Autodesk Inventor part; units mm, degrees
ref_plane "YZ Plane" through (0, 0, 0) normal (1, 0, 0) x (0, 1, 0)
ref_plane "XZ Plane" through (0, 0, 0) normal (0, 1, 0) x (-1, 0, 0)
ref_plane "XY Plane" through (0, 0, 0) normal (0, 0, 1) x (1, 0, 0)
sketch "Skizze1" plane through (0, 0, 0) normal (0, 0, 1) x (1, 0, 0)
  line L0 (0, -63.8443) -> (0, 15.5659)
  line L1 (-61.5828, 0) -> (61.5828, 0)
  line L2 (-13.5, -52.5) -> (13.5, -52.5)
  line L3 (13.5, -52.5) -> (34.4955, -29.2204)
  line L4 (-13.5, -52.5) -> (-34.4955, -29.2204)
  arc A0 (-21.5, 0) -> (-34.4955, -29.2204) centre (-21.5, -17.5) ccw
  arc A1 (34.4955, -29.2204) -> (21.5, 0) centre (21.5, -17.5) ccw
  line L5 (-21.5, 0) -> (21.5, 0)
  point P0 (0, 0)
  dimension "d0" = 43
  dimension "d1" = 27
  dimension "d2" = 35
  dimension "d3" = 17.5
extrude "Extrusion1" add sketch "Skizze1" along normal blind 5
sketch "Skizze2" plane through (0, 0, 5) normal (0, 0, 1) x (1, 0, 0)
  line L0 (-61.5828, 0) -> (61.5828, 0)
  line L1 (0, -63.8443) -> (0, 15.5659)
  arc A0 (-21.5, 0) -> (-34.4955, -29.2204) centre (-21.5, -17.5) ccw
  circle A1 centre (-21.5, -17.5) radius 4
  arc A2 (34.4955, -29.2204) -> (21.5, 0) centre (21.5, -17.5) ccw
  circle A3 centre (21.5, -17.5) radius 10
  circle A4 centre (-11, -42.5) radius 1.7
  circle A5 centre (11, -42.5) radius 1.7
  line L2 (-13.5, -52.5) -> (13.5, -52.5)
  point P0 (0, 0)
  dimension "d7" = 8
  dimension "d8" = 20
  dimension "d9" = 3.4
  dimension "d10" = 3.4
  dimension "d11" = 10
  dimension "d12" = 22
extrude "Extrusion2" cut sketch "Skizze2" against normal up to next
sketch "Skizze3" plane through (0, 0, 5) normal (0, 0, 1) x (1, 0, 0)
  arc A0 (-21.5, 0) -> (-34.4955, -29.2204) centre (-21.5, -17.5) ccw construction
  circle A1 centre (-21.5, -17.5) radius 15 construction
  line L0 (-21.5, -2.5) -> (-21.5, -32.5) construction
  point P0 (0, 0)
  dimension "d15" = 30
hole "Bohrung1" at (-21.5, -32.5, 5) direction (0, 0, -1) diameter 3.5 end up to surface
pattern_circular "Runde Anordnung1" count 3 over 360 about axis through (-21.5, -17.5, 5) along (0, 0, -1) of "Bohrung1"
sketch "Skizze4" plane through (0, 0, 5) normal (0, 0, 1) x (1, 0, 0)
  arc A0 (34.4955, -29.2204) -> (21.5, 0) centre (21.5, -17.5) ccw construction
  circle A1 centre (21.5, -17.5) radius 14 construction
  line L0 (21.5, -3.5) -> (21.5, -31.5) construction
  point P0 (0, 0)
  dimension "d26" = 28
hole "Bohrung2" at (21.5, -31.5, 5) direction (0, 0, -1) diameter 2.459 end up to surface
pattern_circular "Runde Anordnung2" count 6 over 360 about axis through (21.5, -17.5, 5) along (0, 0, -1) of "Bohrung2"
properties part number "Zylinderplatte"
Can you work these out from the model? Positions are in its coordinate system, mm. Round coordinates to 2 decimals unless told otherwise and drop trailing zeros. Loops run counter-clockwise (first coordinate to the right, second up) from the corner with the lowest first, then second, coordinate; pieces in that order, holes last. Notation, with made-up numbers: (80.25, -35.5) -> (110.25, -35.5) arc R11 cw to (110.25, -23.5) -> close; hole circle Ø2 at (30, 24.25). An arc over 180 degrees is marked (long way). Answer in a Markdown table with one row per item.
Item 1: Suppose I cut it at A-A, the plane y = -18.5. List the corners of the cut face in (x, z) for me.
Answer block:
| item | result |
|---|---|
| outline | (-38.97, 0) -> (-25.37, 0) -> (-25.37, 5) -> (-38.97, 5) -> close; (-17.63, 0) -> (11.55, 0) -> (11.55, 5) -> (-17.63, 5) -> close; (31.45, 0) -> (38.97, 0) -> (38.97, 5) -> (31.45, 5) -> close |
Item 2: Suppose I cut it at B-B, the plane x = 23.5. List the corners of the cut face in (y, z) for me.
Answer block:
| item | result |
|---|---|
| outline | (-41.41, 0) -> (-27.3, 0) -> (-27.3, 5) -> (-41.41, 5) -> close; (-7.7, 0) -> (-0.11, 0) -> (-0.11, 5) -> (-7.7, 5) -> close |
Item 3: We'd pull the mould along Y, two halves only. Please class faces 1 (the flat face through (-1, -26, 5)), 2 (the flat face through (0, -52.5, 2)), 3 (the cylindrical face through (34.715, -11.067, 2.465)): released by +Y, released by -Y, zero draft, split by the parting line, or undercut.
Answer block:
| item | result |
|---|---|
| face 1 | zero draft |
| face 2 | released by -Y |
| face 3 | undercut |
Item 4: If I drill on probe 1 along X at (y, z) = (-17, 0.8); probe 2 along X at (y, z) = (-10, 1.8); probe 3 along Y at (x, z) = (21, 2.9), over which ranges is the centre line in solid material (lowest first)?
Answer block:
| item | result |
|---|---|
| probe 1 | -38.99 to -25.47, -17.53 to 11.51, 31.49 to 38.99 |
| probe 2 | -37.31 to -36.24, -32.74 to -10.26, -6.76 to 8.25, 10.5 to 14.89, 28.11 to 32.5, 34.75 to 37.31 |
| probe 3 | -44.18 to -32.62, -30.38 to -27.49, -7.51 to -4.62, -2.38 to 0 |
Item 5: Suppose I cut it at D-D, the plane y = -10.5. List the corners of the cut face in (x, z) for me, plus the area to 3 significant figures.
Answer block:
| item | result |
|---|---|
| outline | (-37.54, 0) -> (-36.17, 0) -> (-36.17, 5) -> (-37.54, 5) -> close; (-32.81, 0) -> (-10.19, 0) -> (-10.19, 5) -> (-32.81, 5) -> close; (-6.83, 0) -> (8.15, 0) -> (8.15, 5) -> (-6.83, 5) -> close; (10.61, 0) -> (14.36, 0) -> (14.36, 5) -> (10.61, 5) -> close; (28.64, 0) -> (32.39, 0) -> (32.39, 5) -> (28.64, 5) -> close; (34.85, 0) -> (37.54, 0) -> (37.54, 5) -> (34.85, 5) -> close |
| area | 246 mm² |
Item 6: Suppose I cut it at C-C, the plane z = 2.4. Give the number of separate pieces and of enclosed holes in the cut face, plus the area to 3 significant figures.
Answer block:
| item | result |
|---|---|
| separate pieces | 1 |
| enclosed holes | 13 |
| area | 2,790 mm² |
Item 7: Will these pins go through, and if not, where does the flat tip stop? P1, Ø3, axis at y = -42.5, z = 0.5, coming from the -X side; P2, Ø2, axis at y = -26, z = 1, coming from the +X side; P3, Ø1.5, axis at y = -22, z = 4, coming from the +X side.
Answer block:
| item | result |
|---|---|
| P1 | x = -23.87 |
| P2 | x = 37.31 |
| P3 | x = 38.59 |
